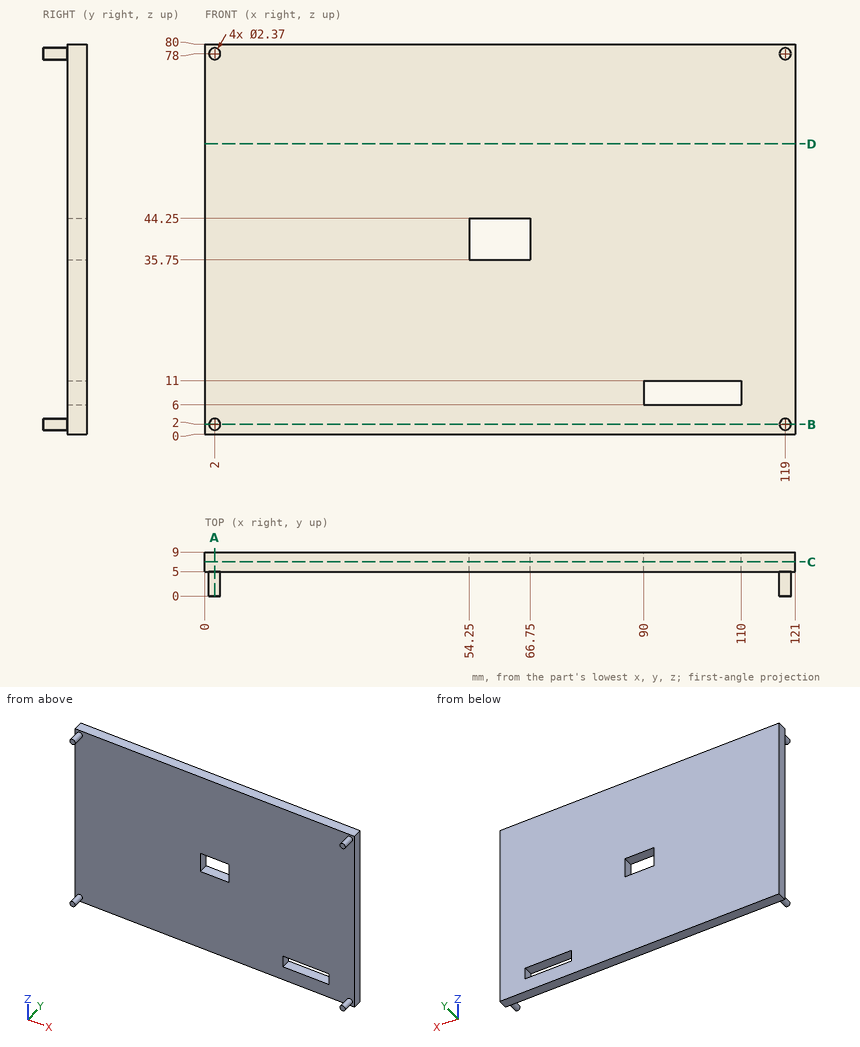
Check sheet for the drawn part. Datum: minimum x, y, z corner. Units: mm. Give positions to 0.01 mm unless a question says otherwise; leave off trailing zeros. Write each loop counter-clockwise with the first axis right and the second up, starting at its lowest first coordinate (ties: lowest second). Pieces come first, ordered by that corner, then holes.
(1) Cross-section at B-B (z = 2). Enter the section's corners in (x, y) (3 decimals), plus the area to 3 significant figures.
(2) Cross-section at D-D (z = 59.5). Enter the section's corners in (x, y), plus the area to 3 significant figures.
(3) Material ranges on line 1 (Z direction, x = 99, y = 7.75); line 2 (Y direction, x = 99, z = 74); line 3 (X direction, y = 8.5, z = 43), recorded low to high.
(4) Cross-section at A-A (x = 2). Enter the section's corners in (y, z) (3 decimals).
(5) Cross-section at C-C (y = 7). Enter the section's corners in (x, z).
(6) Gauge pin test, flat ends, axial feed: pin 1 (2 mm diameter, centred on x = 60.5, y = 6.5, fed in from -Z); pin 2 (24 mm diameter, centred on x = 50.5, z = 51.5, fed in from -Y). Record the tip position at first contact, or that the pin passes through.
Worked out:
1. outline: (0, 5) - (0.815, 5) - (0.815, 0) - (3.185, 0) - (3.185, 5) - (117.815, 5) - (117.815, 0) - (120.185, 0) - (120.185, 5) - (121, 5) - (121, 9) - (0, 9) - close
1. area: 508 mm2
2. outline: (0, 5) - (121, 5) - (121, 9) - (0, 9) - close
2. area: 484 mm2
3. line 1: z = 0 to 6, 11 to 80
3. line 2: y = 5 to 9
3. line 3: x = 0 to 54.25, 66.75 to 121
4. outline: (0, 0.815) - (5, 0.815) - (5, 0) - (9, 0) - (9, 80) - (5, 80) - (5, 79.185) - (0, 79.185) - (0, 76.815) - (5, 76.815) - (5, 3.185) - (0, 3.185) - close
5. outline: (0, 0) - (121, 0) - (121, 80) - (0, 80) - close; hole (54.25, 35.75) - (66.75, 35.75) - (66.75, 44.25) - (54.25, 44.25) - close; hole (90, 6) - (110, 6) - (110, 11) - (90, 11) - close
6. pin 1: stops at z = 0
6. pin 2: stops at y = 5
